from build123d import *

# Parameters (mm, degrees)
BOSS_EXTRU_1_DEPTH      = 1.2
ENL_V_START             = -1.2
ENL_V_MAT_EXTRU_1_DEPTH = 1.2
ENL_V_MAT_EXTRU_2_DEPTH = 0.01


with BuildPart() as part:
    # Esquisse1 → Boss.-Extru.1 (new body)
    with BuildSketch(Plane(origin=(0, 0, 0), x_dir=(1, 0, 0), z_dir=(0, 1, 0))):
        with BuildLine():
            Line((-15.75, 11.9), (-12.75, 11.9))
            ThreePointArc((-12.75, 11.9), (-10.842060454, 11.495351769), (-10.238526329, 13.35))
            Line((-10.238526329, 13.35), (15.75, 13.35))
            Line((15.75, 13.35), (15.75, -15.95))
            Line((15.75, -15.95), (-8.85, -15.95))
            Line((-8.85, -15.95), (-8.85, -14.65))
            Line((-8.85, -14.65), (-10.65, -14.65))
            Line((-10.65, -14.65), (-10.65, -13.35))
            Line((-10.65, -13.35), (-15.75, -13.35))
            Line((-15.75, -13.35), (-15.75, 11.9))
        make_face()
    extrude(amount=BOSS_EXTRU_1_DEPTH)

    # Esquisse3 → Enlèv. mat.-Extru.1 (cut)
    with BuildSketch(Plane(origin=(0, 1.2, 0), x_dir=(1, 0, 0), z_dir=(0, 1, 0)).offset(ENL_V_START)):
        with BuildLine():
            Line((-10.112997726, 12.758125458), (-10.112997726, 13.35))
            Line((-10.112997726, 13.35), (-10.238526329, 13.35))
            ThreePointArc((-10.238526329, 13.35), (-10.144725054, 13.060645252), (-10.112997726, 12.758125458))
        make_face()
    extrude(amount=ENL_V_MAT_EXTRU_1_DEPTH, mode=Mode.SUBTRACT)

    # Esquisse4 → Enlèv. mat.-Extru.2 (cut)
    with BuildSketch(Plane(origin=(0, 1.2, 0), x_dir=(1, 0, 0), z_dir=(0, 1, 0))):
        with BuildLine():
            Line((-1.05, 11.35), (4.95, 11.35))
            ThreePointArc((4.95, 11.35), (7.35, 7.55), (4.95, 3.75))
            Line((4.95, 3.75), (-1.05, 3.75))
            ThreePointArc((-1.05, 3.75), (-3.45, 7.55), (-1.05, 11.35))
        make_face()
        with BuildLine():
            Line((-1.05, -7.35), (4.95, -7.35))
            ThreePointArc((4.95, -7.35), (7.35, -11.15), (4.95, -14.95))
            Line((4.95, -14.95), (-1.05, -14.95))
            ThreePointArc((-1.05, -14.95), (-3.45, -11.15), (-1.05, -7.35))
        make_face()
        with BuildLine():
            Line((-9.95, 2), (-3.95, 2))
            ThreePointArc((-3.95, 2), (-1.55, -1.8), (-3.95, -5.6))
            Line((-3.95, -5.6), (-9.95, -5.6))
            ThreePointArc((-9.95, -5.6), (-12.35, -1.8), (-9.95, 2))
        make_face()
        with BuildLine():
            Line((7.55, 1.2), (7.55, -4.8))
            ThreePointArc((7.55, -4.8), (11.35, -7.2), (15.15, -4.8))
            Line((15.15, -4.8), (15.15, 1.2))
            ThreePointArc((15.15, 1.2), (11.35, 3.6), (7.55, 1.2))
        make_face()
    extrude(amount=-ENL_V_MAT_EXTRU_2_DEPTH, mode=Mode.SUBTRACT)


solid = part.part
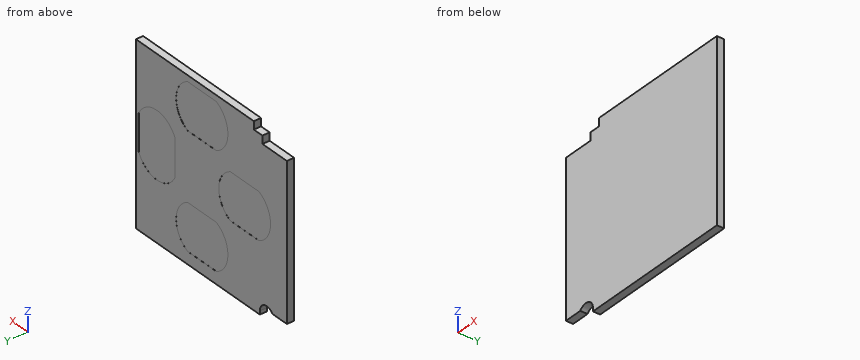
Can you work these out from the model? Positions are in its coordinate system, mm. Coordinates: 2 decimals unless noted, no trailing zeros. Write each loop counter-clockwise with the first axis right and the second up, starting at its lowest first coordinate (ties: lowest second). Pieces come first, ordered by that corner, then holes.
Q1. For P1, Ø2.5, axis at x = -7.5, z = 1, coming from the +Y side, with a flat end and sliding along its axis, tell me the tip position at first contact or that it passes through.
Results found:
P1: stops at y = 1.19
Q2. Imagine slicing it at A-A, the plane y = 0.6. List the corners of the cut face in (x, z) for me.
Results found:
outline: (-15.75, -11.9) - (-12.75, -11.9) arc R1.46 cw to (-10.11, -12.76) - (-10.11, -13.35) - (15.75, -13.35) - (15.75, 15.95) - (-8.85, 15.95) - (-8.85, 14.65) - (-10.65, 14.65) - (-10.65, 13.35) - (-15.75, 13.35) - close
Q3. Please list where these lines run through material, in increasing order: L1, parallel to Y at x = 2.5, z = -8.25; L2, parallel to X at y = 1.05, z = 14; L3, parallel to Z at x = -14, y = 0.75.
Results found:
L1: y = 0 to 1.19
L2: x = -10.65 to 15.75
L3: z = -11.9 to 13.35
